Read the model definition and answer for the solid it produces. Units are mm, in the model's axes. Face numbers are marked on the shaded views. A direction names the side the tool comes from. Round coordinates to 2 decimals unless told otherwise and drop trailing zeros. Order: outer loops, then holes, each group sorted by start corner. A loop starts at its lowest first (then second) coordinate and runs counter-clockwise, first axis right, second up. Notation, with made-up numbers: (38, 51) - (49, 51) arc R5 cw to (49, 58) - close; hole circle Ø11 at (34, 49). An arc over 180 degrees is marked (long way). One line per question, with ' | ' between items. Start each with the question number.
1) The part is cut by section B-B, the plane z = 12.5. Give the vertices of the cut face in (x, y), plus the area to 3 significant figures.
2) The part is cut by section C-C, the plane x = 23.5. Give the vertices of the cut face in (y, z), plus the area to 3 significant figures.
3) Straight lines are drawn through the part: line 1 (Y direction, x = 0, z = 17); line 2 (X direction, y = 26.5, z = 7.25); line 3 (X direction, y = 0, z = 0.8). For each, find the intervals that lie inside material, in ascending order. Write a range as from..to.
4) The mould has two halves that part along Y. Classify the marked faces 1, 2 and 3: pulls with the +Y half, pulls with the -Y half, needs draft (parallel to the pull), parting line crosses it, or undercut.
5) Flat-ended cylindrical pins translate along their axes: pin 1 (2 mm diameter, centred on x = 28, y = -16.5, fed in from +Z); pin 2 (5 mm diameter, centred on y = -25, z = 2.5, fed in from -X); pin 3 (10 mm diameter, centred on y = 25.5, z = 14.5, fed in from -X); pin 4 (8 mm diameter, centred on x = -23.5, y = -16.5, fed in from -Z). Find the tip coordinate at first contact, or state that the pin passes through.
6) For the marked faces 4, 5 and 6, determine the directions among +Z, -Z, +X, -X, +Y, -Y from which every point of the face is accessible in a straight line to the end or side of a thin tool.
7) The part is cut by section D-D, the plane y = 29.5. Give the vertices of the cut face in (x, z).
8) The part is cut by section A-A, the plane x = 0. Give the vertices of the cut face in (y, z).
from build123d import *

# Parameters (mm, degrees)
F0_R      = 42
F1_DEPTH  = 9
F2_R      = 42
F2_R_2    = 20
F3_DEPTH  = 3
F4_R      = 15
F5_DEPTH  = 15
F8_DEPTH  = 25
F9_R      = 5
F10_DEPTH = 24.001
F11_D     = 17.5
F11_DEPTH = 20
F11_TIP   = 5.2575304165


with BuildPart() as f1:
    # F0 (on Top) → F1 (new body)
    with BuildSketch(Plane.XY):
        Circle(F0_R)
    extrude(amount=F1_DEPTH)

    # F2 (on face) → F3 (cut)
    with BuildSketch(Plane(origin=(0, 0, 0), x_dir=(1, 0, 0), z_dir=(0, 0, -1))):
        Circle(F2_R)
        Circle(F2_R_2, mode=Mode.SUBTRACT)
    extrude(amount=-F3_DEPTH, mode=Mode.SUBTRACT)

    # F4 (on face) → F5 (join)
    with BuildSketch(Plane.XY.offset(9)):
        Circle(F4_R)
    extrude(amount=F5_DEPTH)

    # F7 (on face) → F8 (cut)
    with BuildSketch(Plane.XY.offset(9)):
        with BuildLine():
            ThreePointArc((-3.2963309195, 34.8444285714), (0, 31.7), (3.2963309195, 34.8444285714))
            ThreePointArc((3.2963309195, 34.8444285714), (0, 35), (-3.2963309195, 34.8444285714))
        make_face()
        with BuildLine():
            ThreePointArc((-3.2963309195, 34.8444285714), (0, 35), (3.2963309195, 34.8444285714))
            ThreePointArc((3.2963309195, 34.8444285714), (3.2990826023, 34.9221926553), (3.3, 35))
            ThreePointArc((3.3, 35), (-0.0778073447, 38.2990826023), (-3.2963309195, 34.8444285714))
        make_face()
        with BuildLine():
            ThreePointArc((-21.4487373415, 24.7487373415), (-21.6710068674, 25.9393569822), (-22.3078737832, 26.9695896756))
            ThreePointArc((-22.3078737832, 26.9695896756), (-24.7487373415, 24.7487373415), (-26.9695896756, 22.3078737832))
            ThreePointArc((-26.9695896756, 22.3078737832), (-23.4143484744, 21.7305580309), (-21.4487373415, 24.7487373415))
        make_face()
        with BuildLine():
            ThreePointArc((-26.9695896756, 22.3078737832), (-24.7487373415, 24.7487373415), (-22.3078737832, 26.9695896756))
            ThreePointArc((-22.3078737832, 26.9695896756), (-27.0821897194, 27.0821897194), (-26.9695896756, 22.3078737832))
        make_face()
        with BuildLine():
            ThreePointArc((-31.7, 0), (-32.6121782191, 2.2777855788), (-34.8444285714, 3.2963309195))
            ThreePointArc((-34.8444285714, 3.2963309195), (-35, 0), (-34.8444285714, -3.2963309195))
            ThreePointArc((-34.8444285714, -3.2963309195), (-32.6121782191, -2.2777855788), (-31.7, 0))
        make_face()
        with BuildLine():
            ThreePointArc((-34.8444285714, -3.2963309195), (-35, 0), (-34.8444285714, 3.2963309195))
            ThreePointArc((-34.8444285714, 3.2963309195), (-38.3, 0), (-34.8444285714, -3.2963309195))
        make_face()
        with BuildLine():
            ThreePointArc((-26.9695896756, -22.3078737832), (-27.0821897194, -27.0821897194), (-22.3078737832, -26.9695896756))
            ThreePointArc((-22.3078737832, -26.9695896756), (-24.7487373415, -24.7487373415), (-26.9695896756, -22.3078737832))
        make_face()
        with BuildLine():
            ThreePointArc((-26.9695896756, -22.3078737832), (-24.7487373415, -24.7487373415), (-22.3078737832, -26.9695896756))
            ThreePointArc((-22.3078737832, -26.9695896756), (-21.6710068674, -25.9393569822), (-21.4487373415, -24.7487373415))
            ThreePointArc((-21.4487373415, -24.7487373415), (-23.4143484744, -21.7305580309), (-26.9695896756, -22.3078737832))
        make_face()
        with BuildLine():
            ThreePointArc((-3.2963309195, -34.8444285714), (0, -35), (3.2963309195, -34.8444285714))
            ThreePointArc((3.2963309195, -34.8444285714), (0, -31.7), (-3.2963309195, -34.8444285714))
        make_face()
        with BuildLine():
            ThreePointArc((3.3, -35), (3.2990826023, -34.9221926553), (3.2963309195, -34.8444285714))
            ThreePointArc((3.2963309195, -34.8444285714), (0, -35), (-3.2963309195, -34.8444285714))
            ThreePointArc((-3.2963309195, -34.8444285714), (-0.0778073447, -38.2990826023), (3.3, -35))
        make_face()
        with BuildLine():
            ThreePointArc((28.0487373415, -24.7487373415), (27.7669166522, -23.4143484744), (26.9695896756, -22.3078737832))
            ThreePointArc((26.9695896756, -22.3078737832), (24.7487373415, -24.7487373415), (22.3078737832, -26.9695896756))
            ThreePointArc((22.3078737832, -26.9695896756), (25.9393569822, -27.8264678156), (28.0487373415, -24.7487373415))
        make_face()
        with BuildLine():
            ThreePointArc((22.3078737832, -26.9695896756), (24.7487373415, -24.7487373415), (26.9695896756, -22.3078737832))
            ThreePointArc((26.9695896756, -22.3078737832), (22.4152849636, -22.4152849636), (22.3078737832, -26.9695896756))
        make_face()
        with BuildLine():
            ThreePointArc((34.8444285714, 3.2963309195), (34.9610855095, 1.65), (35, 0))
            ThreePointArc((35, 0), (34.9610855095, -1.65), (34.8444285714, -3.2963309195))
            ThreePointArc((34.8444285714, -3.2963309195), (37.2777855788, -2.3878217809), (38.3, 0))
            ThreePointArc((38.3, 0), (37.2777855788, 2.3878217809), (34.8444285714, 3.2963309195))
        make_face()
        with BuildLine():
            ThreePointArc((34.8444285714, -3.2963309195), (34.9610855095, -1.65), (35, 0))
            ThreePointArc((35, 0), (34.9610855095, 1.65), (34.8444285714, 3.2963309195))
            ThreePointArc((34.8444285714, 3.2963309195), (31.7, 0), (34.8444285714, -3.2963309195))
        make_face()
        with BuildLine():
            ThreePointArc((22.3078737832, 26.9695896756), (22.4152849636, 22.4152849636), (26.9695896756, 22.3078737832))
            ThreePointArc((26.9695896756, 22.3078737832), (24.7487373415, 24.7487373415), (22.3078737832, 26.9695896756))
        make_face()
        with BuildLine():
            ThreePointArc((22.3078737832, 26.9695896756), (24.7487373415, 24.7487373415), (26.9695896756, 22.3078737832))
            ThreePointArc((26.9695896756, 22.3078737832), (27.7669166522, 23.4143484744), (28.0487373415, 24.7487373415))
            ThreePointArc((28.0487373415, 24.7487373415), (25.9393569822, 27.8264678156), (22.3078737832, 26.9695896756))
        make_face()
    extrude(amount=-F8_DEPTH, mode=Mode.SUBTRACT)

    # F9 (on face) → F10 (cut, through all)
    with BuildSketch(Plane(origin=(0, 0, 0), x_dir=(1, 0, 0), z_dir=(0, 0, -1))):
        Circle(F9_R)
    extrude(amount=-F10_DEPTH, mode=Mode.SUBTRACT)

    # F11
    with Locations(Plane.XY.offset(24)):
        with Locations((0, 0)):
            Hole(F11_D / 2, depth=F11_DEPTH)
            with Locations((0, 0, -(F11_DEPTH + F11_TIP / 2))):  # 118° drill point
                Cone(0, F11_D / 2, F11_TIP, mode=Mode.SUBTRACT)


solid = f1.part
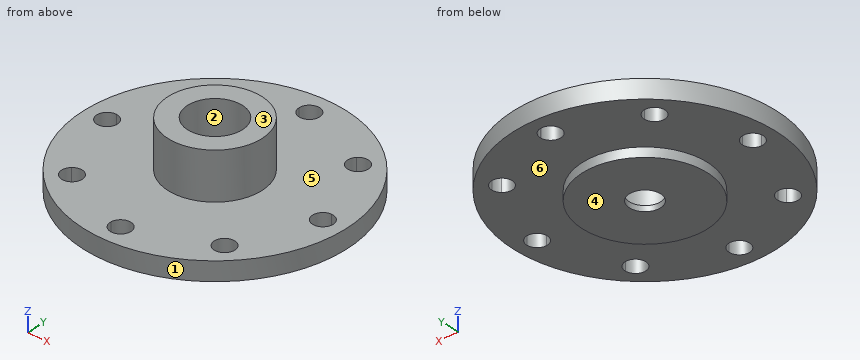
Values:
1) outline: circle Ø30 at (0, 0); hole circle Ø17.5 at (0, 0) | area: 466 mm^2
2) outline: (-34.81, 3) - (-27.8, 3) - (-27.8, 9) - (-34.81, 9) - close; (-21.69, 3) - (21.69, 3) - (21.69, 9) - (-21.69, 9) - close; (27.8, 3) - (34.81, 3) - (34.81, 9) - (27.8, 9) - close | area: 344 mm^2
3) line 1: y = -15..-8.75, 8.75..15 | line 2: x = -32.58..-27.55, -21.95..21.95, 27.55..32.58 | line 3: x = -20..-5, 5..20
4) face 1: parting line crosses it | face 2: undercut | face 3: needs draft
5) pin 1: stops at z = 9 | pin 2: stops at x = -35.43 | pin 3: passes through | pin 4: stops at z = 3
6) face 4: -Z, +X, -X, +Y, -Y | face 5: +Z | face 6: -Z
7) outline: (-29.9, 3) - (29.9, 3) - (29.9, 9) - (-29.9, 9) - close
8) outline: (-42, 3) - (-38.3, 3) - (-38.3, 9) - (-42, 9) - close; (-31.7, 3) - (-20, 3) - (-20, 0) - (-5, 0) - (-5, 1.75) - (-8.75, 4) - (-8.75, 24) - (-15, 24) - (-15, 9) - (-31.7, 9) - close; (5, 0) - (20, 0) - (20, 3) - (31.7, 3) - (31.7, 9) - (15, 9) - (15, 24) - (8.75, 24) - (8.75, 4) - (5, 1.75) - close; (38.3, 3) - (42, 3) - (42, 9) - (38.3, 9) - close
